Could you check a few things on this model? Use its own coordinates, in mm. Face numbers are marked on the shaded views. Round coordinates to 2 decimals unless told otherwise and drop trailing zeros. Write each loop counter-clockwise with the first axis right and the second up, starting at its lowest first coordinate (ties: lowest second). Pieces come first, ordered by that corner, then holes. Notation, with made-up numbers: (75, 60.5) - (91, 60.5) arc R15 ccw to (91, 77.5) - close; hole circle Ø6 at (-29.5, -4). An arc over 180 degrees is marked (long way). Put each result on its own line as item: value.
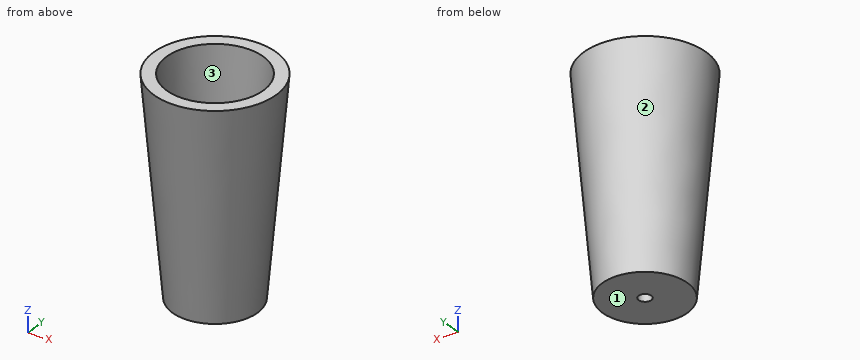
from build123d import *

# Parameters (mm, degrees)
F0_R     = 10
F1_DEPTH = 50
F1_TAPER = -5
F2_T     = -3
F3_DEPTH = 10
F4_D     = 3
F5_R     = 2


with BuildPart() as f1:
    # F0 (on Top) → F1 (new body)
    with BuildSketch(Plane.XY):
        Circle(F0_R)
    extrude(amount=F1_DEPTH, taper=F1_TAPER)

    # F2
    f2_openings = [f1.faces().sort_by_distance(p)[0] for p in [
        (0, 0, 50),
    ]]
    offset(amount=F2_T, openings=f2_openings, kind=Kind.INTERSECTION)

    # F0 (on Top) → F3 (join)
    with BuildSketch(Plane.XY):
        Circle(F0_R)
    extrude(amount=F3_DEPTH)

    # F4 (through all)
    with Locations(Plane(origin=(0, 0, 0), x_dir=(1, 0, 0), z_dir=(0, 0, -1))):
        with Locations((0, 0)):
            Hole(F4_D / 2)

    # F5
    f5_edges = [f1.edges().sort_by_distance(p)[0] for p in [
        (-7.863427, 0, 10),
    ]]
    fillet(f5_edges, radius=F5_R)


solid = f1.part
(1) If we mould it in two halves opening along X, with no side actions, what happens to the marked faces 1, 2 and 3? For each: pulls with the +X half, pulls with the -X half, needs draft (parallel to the pull), parting line crosses it, or undercut.
Values found:
face 1: needs draft
face 2: parting line crosses it
face 3: undercut
(2) Imagine slicing it at C-C, the plane z = 27. List the corners of the cut face in (x, y) for me, then the cut area to 3 significant figures.
Values found:
outline: circle Ø24.72 at (0, 0); hole circle Ø18.7 at (0, 0)
area: 205 mm^2
(3) I'm going to push flat-ended pins straight in: pin 1 (5 mm diameter, centred on x = -2.5, y = -11, fed in from -Z); pin 2 (1.5 mm diameter, centred on y = 10.5, z = 44, fed in from -X); pin 3 (8 mm diameter, centred on y = -10, z = 33.5, fed in from +X); pin 4 (5 mm diameter, centred on x = 1.5, z = 20, fed in from -Y). Where does each tip first touch, or does it pass through?
Values found:
pin 1: stops at z = 0
pin 2: stops at x = -9.84
pin 3: stops at x = 11.49
pin 4: stops at y = -11.94
(4) Imagine slicing it at A-A, the plane x = 0. List the corners of the cut face in (y, z) for me, then the cut area to 3 significant figures.
Values found:
outline: (-14.37, 50) - (-10, 0) - (-1.5, 0) - (-1.5, 10) - (-6.03, 10) arc R2 cw to (-8.02, 11.83) - (-11.36, 50) - close; (1.5, 0) - (10, 0) - (14.37, 50) - (11.36, 50) - (8.02, 11.83) arc R2 cw to (6.03, 10) - (1.5, 10) - close
area: 421 mm^2
(5) Imagine slicing it at B-B, the plane z = 13.5. List the corners of the cut face in (x, y) for me, then the cut area to 3 significant figures.
Values found:
outline: circle Ø22.36 at (0, 0); hole circle Ø16.34 at (0, 0)
area: 183 mm^2
(6) Please list where these lines run through material, in increasing order: probe 1 along Z at (x, y) = (1.5, 3.75); probe 2 along Y at (x, z) = (-6.75, 31); probe 3 along X at (y, z) = (-2, 20). Write a range as from..to.
Values found:
probe 1: z = 0..10
probe 2: y = -10.77..-6.97, 6.97..10.77
probe 3: x = -11.58..-8.51, 8.51..11.58
